Autodesk Inventor part; units mm, degrees
ref_plane "YZ Plane" through (0, 0, 0) normal (1, 0, 0) x (0, 1, 0)
ref_plane "XZ Plane" through (0, 0, 0) normal (0, 1, 0) x (-1, 0, 0)
ref_plane "XY Plane" through (0, 0, 0) normal (0, 0, 1) x (1, 0, 0)
sketch "Sketch1" plane through (0, 0, 0) normal (0, 0, 1) x (1, 0, 0)
  line L0 (-41.3322, 31.5) -> (12.6678, 31.5)
  line L1 (12.6678, 31.5) -> (12.6678, -31.5)
  line L2 (12.6678, -31.5) -> (-41.3322, -31.5)
  line L3 (-41.3322, -31.5) -> (-41.3322, 31.5)
  line L4 (-89.332, 0) -> (29.6678, 0)
  point P0 (0, 0)
  dimension "leveys" = 54
  dimension "pituus" = 63
extrude "Extrusion1" add sketch "Sketch1" along normal blind 1
sketch "Sketch2" plane through (0, 0, 1) normal (0, 0, 1) x (1, 0, 0)
  line L0 (12.6678, 31.5) -> (-41.3322, 31.5)
  line L1 (-41.3322, -31.5) -> (12.6678, -31.5)
  line L2 (12.6678, 31.5) -> (11.6678, 31.5)
  line L3 (11.6678, 31.5) -> (11.6678, -31.5)
  line L4 (11.6678, -31.5) -> (12.6678, -31.5)
  line L5 (12.6678, -31.5) -> (12.6678, 31.5)
  line L6 (11.6678, 30.5) -> (-41.3322, 30.5)
  line L7 (-41.3322, 31.5) -> (-41.3322, -31.5)
  line L8 (-41.3322, -30.5) -> (11.6678, -30.5)
  point P0 (0, 0)
  dimension "d4" = 1
  dimension "laita" = 1
  dimension "d9" = 1
extrude "Extrusion2" add sketch "Sketch2" along normal blind 40 contours L5 L1 L3 L0
sketch "Sketch3" plane through (12.6678, -31.5, 0) normal (1, 0, 0) x (0, 0, -1)
  circle A0 centre (-10.9634, 31.5) radius 5
  line L0 (-41, 0) -> (-41, 63)
  line L1 (-41, 31.5) -> (34.5285, 31.5) construction
  line L2 (-1, 63) -> (-1, 0)
  circle A1 centre (-19.1022, 49) radius 2.1
  circle A2 centre (-19.1022, 14) radius 2.1
  point P0 (0, 31.5)
  dimension "d7" = 10
  dimension "PIKKU" = 4.2
  dimension "d13" = 4.2
  dimension "d14" = 19.3
  dimension "d16" = 35
extrude "Extrusion3" cut sketch "Sketch3" against normal up to next
sketch "Sketch4" plane through (-41.3322, 31.5, 0) normal (0, 1, 0) x (1, 0, 0)
  line L0 (0, 0) -> (54, 0)
  line L1 (54, 0) -> (0, 0)
  line L2 (0, 0) -> (0, -21)
  line L3 (0, -21) -> (31, -21)
  line L4 (54, -22.5156) -> (54, 0)
  line L5 (54, 0) -> (54, -41)
  line L6 (54, -41) -> (31, -41)
  line L7 (31, -41) -> (31, -21)
  line L8 (54, -22.5156) -> (54, -41)
  point P0 (41.3322, 0)
  dimension "d24" = 20
  dimension "d25" = 23
extrude "Extrusion4" add sketch "Sketch4" along normal blind 1
mirror "Mirror1" about plane through (0, 0, 0) normal (0, 1, 0) of "Extrusion4"
sketch "Sketch7" plane through (0, 0, 0) normal (0, 0, -1) x (-1, 0, 0)
  line L0 (-12.6678, 30) -> (41.3322, 30)
  line L1 (-12.6678, -30) -> (41.3322, -30)
  line L2 (89.332, 0) -> (-29.6678, 0)
  line L3 (41.3322, -32.5) -> (41.3322, 32.5)
  line L4 (-12.6678, 32.5) -> (-12.6678, -32.5)
  line L5 (-12.6678, -32.5) -> (41.3322, -32.5)
  line L6 (-12.6678, 32.5) -> (41.3322, 32.5)
  point P0 (0, 0)
  dimension "d30" = 60
extrude "Extrusion7" add sketch "Sketch7" along normal blind 5 contours L4 L6 L3 L0 | L1 L3 L5 L4
equation "\"d4\" = laita"
equation "\"d9\" = laita"
equation "\"d13\" = PIKKU"
properties part number "ProjectXBase"
Can you work these out from the model? Positions are in its coordinate system, mm. A direction names the side the tool comes from. Coordinates: 2 decimals unless noted, no trailing zeros. Write each loop counter-clockwise with the first axis right and the second up, starting at its lowest first coordinate (ties: lowest second). Pieces come first, ordered by that corner, then holes. Notation, with made-up numbers: M 52.25,45 L 84.25,45 A4 cw 84.25,49 Z; hole C 16.25,3.25 d1. An arc over 180 degrees is marked long. Answer as CSV lines item,"result".
Item 1: Imagine slicing it at D-D on y = 22. List the corners of the cut face in (x, z) for me.
Geometry results:
outline,"M -41.33,0 L 12.67,0 L 12.67,41 L 11.67,41 L 11.67,1 L -41.33,1 Z"
Item 2: Imagine slicing it at B-B on x = -17. List the corners of the cut face in (y, z) for me, plus the area to 3 significant figures.
Geometry results:
outline,"M -32.5,-5 L -30,-5 L -30,0 L 30,0 L 30,-5 L 32.5,-5 L 32.5,21 L 31.5,21 L 31.5,1 L -31.5,1 L -31.5,21 L -32.5,21 Z"
area,"130 mm2"
Item 3: On a 3-axis mill with a long thin cutter (end or side, diameter ignored), from which of +Z, -Z, +X, -X, +Y, -Y can I reach the whole of each face in a straight line? I mean faces 1 (the flat face through (-41.332, 0.2, 0.4)), 2 (the flat face through (-15, 0, 1)), 3 (the flat face through (-14, 30, -2)). Say none if no direction works.
Geometry results:
face 1,"+Z, -Z, -X, +Y, -Y"
face 2,"+Z, -X"
face 3,"-Z, +X, -X"
Item 4: I'm going to push flat-ended pins straight in: P1, Ø1.5, axis at x = -33, y = -20, coming from the -Z side; P2, Ø0.5, axis at y = -32, z = 33.5, coming from the -X side; P3, Ø0.5, axis at x = -22, y = 32, coming from the +Z side; P4, Ø9, axis at y = 0, z = 10.96, coming from the -X side. Where does each tip first touch, or does it pass through?
Geometry results:
P1,"stops at z = 0"
P2,"stops at x = -10.33"
P3,"stops at z = 21"
P4,"passes through"
Item 5: We'd pull the mould along Z, two halves only. Please class faces 4 (the cylindrical face through (12.17, -16.08, 20.65)), 5 (the flat face through (-14, 31, -5)), 6 (the cylindrical face through (12.17, 18.92, 20.65)), 7 (the flat face through (12.668, 0, 23)): +Z half, -Z half, draft (parallel to the pull), parting line (faces both ways), or undercut.
Geometry results:
face 4,"undercut"
face 5,"-Z half"
face 6,"undercut"
face 7,"draft"
Item 6: Please list where these lines run through material, in increasing order: line 1 along Y through (x, z) = (9.5, 14.5); line 2 along X through (y, z) = (-5, 18); line 3 along Z through (x, y) = (1, -20.5).
Geometry results:
line 1,"y = -32.5 to -31.5, 31.5 to 32.5"
line 2,"x = 11.67 to 12.67"
line 3,"z = 0 to 1"
Item 7: Imagine slicing it at C-C on z = 11.5. List the corners of the cut face in (x, y) for me, plus the area to 3 significant figures.
Geometry results:
outline,"M -41.33,-32.5 L 12.67,-32.5 L 12.67,-4.97 L 11.67,-4.97 L 11.67,-31.5 L -41.33,-31.5 Z; M -41.33,31.5 L 11.67,31.5 L 11.67,4.97 L 12.67,4.97 L 12.67,32.5 L -41.33,32.5 Z"
area,"161 mm2"
Item 8: Imagine slicing it at A-A on y = -17.5. List the corners of the cut face in (x, z) for me, plus the area to 3 significant figures.
Geometry results:
outline,"M -41.33,0 L 12.67,0 L 12.67,17 L 11.67,17 L 11.67,1 L -41.33,1 Z; M 11.67,21.2 L 12.67,21.2 L 12.67,41 L 11.67,41 Z"
area,"89.8 mm2"
